from build123d import *

# Parameters (mm, degrees)
SKETCH_1_W          = 30
SKETCH_1_H          = 10
SKETCH_1_W_2        = 26
SKETCH_1_H_2        = 6
EXTRUDE_1_DEPTH     = 45
SKETCH_2_R          = 1.5
CUT_EXTRUDE_1_DEPTH = 49.476798574


with BuildPart() as part:
    # 草图1 → 凸台-拉伸1 (new, symmetric)
    with BuildSketch(Plane(origin=(0, 0, 0), x_dir=(1, 0, 0), z_dir=(0, 1, 0))):
        Rectangle(SKETCH_1_W, SKETCH_1_H)
        Rectangle(SKETCH_1_W_2, SKETCH_1_H_2, mode=Mode.SUBTRACT)
    extrude(amount=EXTRUDE_1_DEPTH, both=True)

    # 草图2 → 切除-拉伸1 (cut, through all)
    with BuildSketch(Plane.XY.offset(5)):
        with Locations((5, 40)):
            Circle(SKETCH_2_R)
        with Locations((10, 5)):
            Circle(SKETCH_2_R)
        Circle(SKETCH_2_R)
        with Locations((-10, 5)):
            Circle(SKETCH_2_R)
        with Locations((-5, 40)):
            Circle(SKETCH_2_R)
        with Locations((5, -30)):
            Circle(SKETCH_2_R)
        with Locations((-5, -30)):
            Circle(SKETCH_2_R)
        with Locations((-10, -40)):
            Circle(SKETCH_2_R)
        with Locations((0, -40)):
            Circle(SKETCH_2_R)
        with Locations((10, -40)):
            Circle(SKETCH_2_R)
    extrude(amount=-CUT_EXTRUDE_1_DEPTH, mode=Mode.SUBTRACT)


solid = part.part
Can you work these out from the model? Positions are in its coordinate system, mm. Coordinates: 2 decimals unless noted, no trailing zeros. Write each loop counter-clockwise with the first axis right and the second up, starting at its lowest first coordinate (ties: lowest second). Pieces come first, ordered by that corner, then holes. Notation, with made-up numbers: (89, -8) -> (131, -8) arc R17 cw to (131, 3) -> close; hole circle Ø11 at (21, 7). An arc over 180 degrees is marked (long way). Write each question's results on one line, items separated by ' | '. Start each with the question number.
Item 1: I'm going to push flat-ended pins straight in: P1, Ø2.5, axis at x = -10, y = -40, coming from the +Z side; P2, Ø4, axis at x = -5, y = -30, coming from the +Z side. Where does each tip first touch, or does it pass through?
Item 2: Thinking about a two-plate mould opening in X: for faces 1 (the flat face through (3, 1, 3)), 2 (the flat face through (-13, 1, 0)), 3 (the flat face through (-15, 1, 0)), 4 (the flat face through (-0.2, -45, -3.4)), which applies, released by +X, released by -X, zero draft, split by the parting line, or undercut?
Item 3: Please list where these lines run through material, in increasing order: probe 1 along Y at (x, z) = (5, -4.1); probe 2 along X at (y, z) = (25, -2.75); probe 3 along Y at (x, z) = (-10, -4.2).
Item 4: If we section it at C-C, the plane x = 5: Write out the boundary of the cut face in (y, z).
Item 5: If we section it at A-A, the plane z = -1: Write out the boundary of the cut face in (x, y), and give its area (3 significant figures).
Item 6: If we section it at B-B, the plane y = -40: Count the separate pieces of the cut face and the enclosed holes in it, and give its area (3 significant figures).
Item 7: If we section it at D-D, the plane y = -30: Write out the boundary of the cut face in (x, z).
Answer block:
1) P1: through | P2: z = 5
2) face 1: undercut | face 2: undercut | face 3: released by -X | face 4: zero draft
3) probe 1: -45 to -31.5, -28.5 to 38.5, 41.5 to 45 | probe 2: -15 to -13, 13 to 15 | probe 3: -45 to -41.5, -38.5 to 3.5, 6.5 to 45
4) outline: (-45, -5) -> (-31.5, -5) -> (-31.5, -3) -> (-45, -3) -> close; (-45, 3) -> (-31.5, 3) -> (-31.5, 5) -> (-45, 5) -> close; (-28.5, -5) -> (38.5, -5) -> (38.5, -3) -> (-28.5, -3) -> close; (-28.5, 3) -> (38.5, 3) -> (38.5, 5) -> (-28.5, 5) -> close; (41.5, -5) -> (45, -5) -> (45, -3) -> (41.5, -3) -> close; (41.5, 3) -> (45, 3) -> (45, 5) -> (41.5, 5) -> close
5) outline: (-15, -45) -> (-13, -45) -> (-13, 45) -> (-15, 45) -> close; (13, -45) -> (15, -45) -> (15, 45) -> (13, 45) -> close | area: 360 mm²
6) separate pieces: 6 | enclosed holes: 0 | area: 108 mm²
7) outline: (-15, -5) -> (-6.5, -5) -> (-6.5, -3) -> (-13, -3) -> (-13, 3) -> (-6.5, 3) -> (-6.5, 5) -> (-15, 5) -> close; (-3.5, -5) -> (3.5, -5) -> (3.5, -3) -> (-3.5, -3) -> close; (-3.5, 3) -> (3.5, 3) -> (3.5, 5) -> (-3.5, 5) -> close; (6.5, -5) -> (15, -5) -> (15, 5) -> (6.5, 5) -> (6.5, 3) -> (13, 3) -> (13, -3) -> (6.5, -3) -> close
